```python
from build123d import *

# Parameters (mm, degrees)
BOSS_EXTRUDE1_DEPTH = 10
SKETCH6_R           = 5
CUT_EXTRUDE1_DEPTH  = 10
SKETCH6_4_R         = 5
CUT_EXTRUDE4_DEPTH  = 10


with BuildPart() as part:
    # Sketch2 → Boss-Extrude1 (new body)
    with BuildSketch(Plane.XY):
        with BuildLine():
            Line((10, 0), (170, 0))
            ThreePointArc((170, 0), (177.071067812, -2.928932188), (180, -10))
            Line((180, -10), (180, -65))
            ThreePointArc((180, -65), (177.071067812, -72.071067812), (170, -75))
            Line((170, -75), (10, -75))
            ThreePointArc((10, -75), (2.928932188, -72.071067812), (0, -65))
            Line((0, -65), (0, -10))
            ThreePointArc((0, -10), (2.928932188, -2.928932188), (10, 0))
        make_face()
    extrude(amount=BOSS_EXTRUDE1_DEPTH)

    # Sketch6 → Cut-Extrude1 (cut)
    with BuildSketch(Plane.XY):
        with Locations((15, -15)):
            Circle(SKETCH6_R)
    extrude(amount=CUT_EXTRUDE1_DEPTH, mode=Mode.SUBTRACT)

    # Sketch6_4 → Cut-Extrude4 (cut)
    with BuildSketch(Plane.XY):
        with Locations(Location((165, -15, 0), (0, 0, 180))):
            Circle(SKETCH6_4_R)
        with Locations(Location((15, -60, 0), (0, 0, 180))):
            Circle(SKETCH6_4_R)
        with Locations((165, -60)):
            Circle(SKETCH6_4_R)
    extrude(amount=CUT_EXTRUDE4_DEPTH, mode=Mode.SUBTRACT)


solid = part.part
```
Input: part model. Units: mm. Frame: model coordinates. Coordinates: 2 decimals unless noted, no trailing zeros. Write each loop counter-clockwise with the first axis right and the second up, starting at its lowest first coordinate (ties: lowest second). Pieces come first, ordered by that corner, then holes. Notation, with made-up numbers: (65.5, -35.75) -> (79.5, -35.75) arc R20 ccw to (79.5, -31.75) -> close; hole circle Ø9 at (-19.75, 0). An arc over 180 degrees is marked (long way). Answer as a JSON object with one key per item and string values.
1. Material intervals for line 1 (Y direction, x = 15, z = 3); line 2 (Y direction, x = 162, z = 1.75); line 3 (X direction, y = -16.5, z = 9), sorted ascending. Write a range as from..to.
Result set:
{"line 1": "y = -75..-65, -55..-20, -10..0", "line 2": "y = -75..-64, -56..-19, -11..0", "line 3": "x = 0..10.23, 19.77..160.23, 169.77..180"}
2. Section C-C on x = 165. Return the cut outline in (y, z), then the cut area to 3 significant figures.
Result set:
{"outline": "(-75, 0) -> (-65, 0) -> (-65, 10) -> (-75, 10) -> close; (-55, 0) -> (-20, 0) -> (-20, 10) -> (-55, 10) -> close; (-10, 0) -> (0, 0) -> (0, 10) -> (-10, 10) -> close", "area": "550 mm2"}
3. Section A-A on y = -18. Return the cut outline in (x, z), then the cut area to 3 significant figures.
Result set:
{"outline": "(0, 0) -> (11, 0) -> (11, 10) -> (0, 10) -> close; (19, 0) -> (161, 0) -> (161, 10) -> (19, 10) -> close; (169, 0) -> (180, 0) -> (180, 10) -> (169, 10) -> close", "area": "1,640 mm2"}
4. Mould query, pull axis Y, two halves, no side actions, for faces 1 (the face through (0, -38, 5)), 2 (the face through (169, -12, 5)), 3 (the face through (177.15, -71.99, 4.93)), 4 (the face through (89, 0, 5)). Classes: released by +Y, released by -Y, zero draft, split by the parting line, or undercut.
Result set:
{"face 1": "zero draft", "face 2": "undercut", "face 3": "released by -Y", "face 4": "released by +Y"}
5. Section B-B on z = 7. Return the cut outline in (x, y).
Result set:
{"outline": "(0, -65) arc R10 ccw to (10, -75) -> (170, -75) arc R10 ccw to (180, -65) -> (180, -10) arc R10 ccw to (170, 0) -> (10, 0) arc R10 ccw to (0, -10) -> close; hole circle Ø10 at (15, -60); hole circle Ø10 at (15, -15); hole circle Ø10 at (165, -60); hole circle Ø10 at (165, -15)"}
6. First-contact query: P1, Ø6, axis at x = 15, y = -15, coming from the -Z side. Flat tip, straight axial feed; report the tip coordinate or a pass-through.
Result set:
{"P1": "passes through"}
